Build history of the part. All positions in model axes, mm. A direction names the side the tool comes from. Give positions to 0.01 mm unless a question says otherwise; leave off trailing zeros. Loops run counter-clockwise (first coordinate to the right, second up) from the corner with the lowest first, then second, coordinate; pieces in that order, holes last. Notation, with made-up numbers: M 79,66.5 L 125,66.5 A24 ccw 125,105.5 Z; hole C 63.25,1.25 d1. An arc over 180 degrees is marked long. Put each result on its own line as item: value.
```python
from build123d import *

# Parameters (mm, degrees)
SKETCH_1_R          = 1.5
SKETCH_1_R_2        = 7.5
EXTRUDE_1_DEPTH     = 2.5
SKETCH_2_W          = 200
SKETCH_2_H          = 2.5
EXTRUDE_2_DEPTH     = 22.5
CUT_EXTRUDE_1_REACH = 327.01
SKETCH_3_R          = 1.5
CUT_EXTRUDE_2_REACH = 238.725
SKETCH_6_R          = 1.5
CUT_EXTRUDE_3_REACH = 303.968
SKETCH_7_R          = 1.5


with BuildPart() as part:
    # Эскиз1 → Бобышка-Вытянуть1 (new body)
    with BuildSketch(Plane.XY):
        Polygon((0, 0), (21, 36.373066959), (221, 36.373066959), (242, 0), (142, -173.205080757), (100, -173.205080757), align=None)
        with Locations((21.48120212, 11.846533479)):
            Circle(SKETCH_1_R, mode=Mode.SUBTRACT)
        with Locations((41.48120212, 11.846533479)):
            Circle(SKETCH_1_R, mode=Mode.SUBTRACT)
        with Locations((31.48120212, -5.473974596)):
            Circle(SKETCH_1_R, mode=Mode.SUBTRACT)
        with Locations((200.51879788, 11.846533479)):
            Circle(SKETCH_1_R, mode=Mode.SUBTRACT)
        with Locations((220.51879788, 11.846533479)):
            Circle(SKETCH_1_R, mode=Mode.SUBTRACT)
        with Locations((210.51879788, -5.473974596)):
            Circle(SKETCH_1_R, mode=Mode.SUBTRACT)
        with Locations((111, -143.204572681)):
            Circle(SKETCH_1_R, mode=Mode.SUBTRACT)
        with Locations((131, -143.204572681)):
            Circle(SKETCH_1_R, mode=Mode.SUBTRACT)
        with Locations((121, -160.525080757)):
            Circle(SKETCH_1_R, mode=Mode.SUBTRACT)
        with Locations((121, -45.610671266)):
            Circle(SKETCH_1_R_2, mode=Mode.SUBTRACT)
    extrude(amount=EXTRUDE_1_DEPTH)

    # Эскиз2 → Бобышка-Вытянуть2 (add)
    with BuildSketch(Plane(origin=(0, 0, 0), x_dir=(-1, 0, 0), z_dir=(0, 0, -1))):
        Polygon((0, 0), (2.165063509, -1.25), (-97.834936491, -174.455080757), (-100, -173.205080757), align=None)
        with Locations((-121, 37.623066959)):
            Rectangle(SKETCH_2_W, SKETCH_2_H)
        Polygon((-242, 0), (-244.165063509, -1.25), (-144.165063509, -174.455080757), (-142, -173.205080757), align=None)
    extrude(amount=-EXTRUDE_2_DEPTH)

    # Эскиз3 → Вырез-Вытянуть1 (cut, up to next)
    with BuildSketch(Plane(origin=(0, 38.873066959, 0), x_dir=(1, 0, 0), z_dir=(0, 1, 0)), mode=Mode.PRIVATE) as cut_extrude_1_sk1:
        with Locations(Location((211, -11.25, 0), (0, 0, 180))):
            Circle(SKETCH_3_R)
    cut_extrude_1_tool1 = extrude(cut_extrude_1_sk1.sketch, amount=-CUT_EXTRUDE_1_REACH, mode=Mode.PRIVATE) & part.part
    # Эскиз3 → Вырез-Вытянуть1 (cut, up to next)
    with BuildSketch(Plane(origin=(0, 38.873066959, 0), x_dir=(1, 0, 0), z_dir=(0, 1, 0)), mode=Mode.PRIVATE) as cut_extrude_1_sk2:
        with Locations(Location((201, -11.25, 0), (0, 0, 180))):
            Circle(SKETCH_3_R)
    cut_extrude_1_tool2 = extrude(cut_extrude_1_sk2.sketch, amount=-CUT_EXTRUDE_1_REACH, mode=Mode.PRIVATE) & part.part
    # Эскиз3 → Вырез-Вытянуть1 (cut, up to next)
    with BuildSketch(Plane(origin=(0, 38.873066959, 0), x_dir=(1, 0, 0), z_dir=(0, 1, 0)), mode=Mode.PRIVATE) as cut_extrude_1_sk3:
        with Locations(Location((41, -11.25, 0), (0, 0, 180))):
            Circle(SKETCH_3_R)
    cut_extrude_1_tool3 = extrude(cut_extrude_1_sk3.sketch, amount=-CUT_EXTRUDE_1_REACH, mode=Mode.PRIVATE) & part.part
    # Эскиз3 → Вырез-Вытянуть1 (cut, up to next)
    with BuildSketch(Plane(origin=(0, 38.873066959, 0), x_dir=(1, 0, 0), z_dir=(0, 1, 0)), mode=Mode.PRIVATE) as cut_extrude_1_sk4:
        with Locations(Location((31, -11.25, 0), (0, 0, 180))):
            Circle(SKETCH_3_R)
    cut_extrude_1_tool4 = extrude(cut_extrude_1_sk4.sketch, amount=-CUT_EXTRUDE_1_REACH, mode=Mode.PRIVATE) & part.part
    add(cut_extrude_1_tool1.solids().sort_by_distance((211, 38.873067, 11.25))[0], mode=Mode.SUBTRACT)
    add(cut_extrude_1_tool2.solids().sort_by_distance((201, 38.873067, 11.25))[0], mode=Mode.SUBTRACT)
    add(cut_extrude_1_tool3.solids().sort_by_distance((41, 38.873067, 11.25))[0], mode=Mode.SUBTRACT)
    add(cut_extrude_1_tool4.solids().sort_by_distance((31, 38.873067, 11.25))[0], mode=Mode.SUBTRACT)

    # Эскиз6 → Вырез-Вытянуть2 (cut, up to next)
    with BuildSketch(Plane(origin=(183.665063509, -106.039073858, 0), x_dir=(0, 0, -1), z_dir=(0.8660254037844386, -0.5000000000000003, 0)), mode=Mode.PRIVATE) as cut_extrude_2_sk1:
        with Locations(Location((-11.25, 111, 0), (0, 0, 90))):
            Circle(SKETCH_6_R)
    cut_extrude_2_tool1 = extrude(cut_extrude_2_sk1.sketch, amount=-CUT_EXTRUDE_2_REACH, mode=Mode.PRIVATE) & part.part
    # Эскиз6 → Вырез-Вытянуть2 (cut, up to next)
    with BuildSketch(Plane(origin=(183.665063509, -106.039073858, 0), x_dir=(0, 0, -1), z_dir=(0.8660254037844386, -0.5000000000000003, 0)), mode=Mode.PRIVATE) as cut_extrude_2_sk2:
        with Locations(Location((-11.25, 101, 0), (0, 0, 90))):
            Circle(SKETCH_6_R)
    cut_extrude_2_tool2 = extrude(cut_extrude_2_sk2.sketch, amount=-CUT_EXTRUDE_2_REACH, mode=Mode.PRIVATE) & part.part
    # Эскиз6 → Вырез-Вытянуть2 (cut, up to next)
    with BuildSketch(Plane(origin=(183.665063509, -106.039073858, 0), x_dir=(0, 0, -1), z_dir=(0.8660254037844386, -0.5000000000000003, 0)), mode=Mode.PRIVATE) as cut_extrude_2_sk3:
        with Locations(Location((-11.25, -59, 0), (0, 0, 90))):
            Circle(SKETCH_6_R)
    cut_extrude_2_tool3 = extrude(cut_extrude_2_sk3.sketch, amount=-CUT_EXTRUDE_2_REACH, mode=Mode.PRIVATE) & part.part
    # Эскиз6 → Вырез-Вытянуть2 (cut, up to next)
    with BuildSketch(Plane(origin=(183.665063509, -106.039073858, 0), x_dir=(0, 0, -1), z_dir=(0.8660254037844386, -0.5000000000000003, 0)), mode=Mode.PRIVATE) as cut_extrude_2_sk4:
        with Locations(Location((-11.25, -69, 0), (0, 0, 90))):
            Circle(SKETCH_6_R)
    cut_extrude_2_tool4 = extrude(cut_extrude_2_sk4.sketch, amount=-CUT_EXTRUDE_2_REACH, mode=Mode.PRIVATE) & part.part
    add(cut_extrude_2_tool1.solids().sort_by_distance((239.165064, -9.910254, 11.25))[0], mode=Mode.SUBTRACT)
    add(cut_extrude_2_tool2.solids().sort_by_distance((234.165064, -18.570508, 11.25))[0], mode=Mode.SUBTRACT)
    add(cut_extrude_2_tool3.solids().sort_by_distance((154.165064, -157.134573, 11.25))[0], mode=Mode.SUBTRACT)
    add(cut_extrude_2_tool4.solids().sort_by_distance((149.165064, -165.794827, 11.25))[0], mode=Mode.SUBTRACT)

    # Эскиз7 → Вырез-Вытянуть3 (cut, up to next)
    with BuildSketch(Plane(origin=(-2.165063509, -1.25, 0), x_dir=(0, 0, 1), z_dir=(-0.8660254037844386, -0.5000000000000003, 0)), mode=Mode.PRIVATE) as cut_extrude_3_sk1:
        with Locations(Location((11.25, -10, 0), (0, 0, 270))):
            Circle(SKETCH_7_R)
    cut_extrude_3_tool1 = extrude(cut_extrude_3_sk1.sketch, amount=-CUT_EXTRUDE_3_REACH, mode=Mode.PRIVATE) & part.part
    # Эскиз7 → Вырез-Вытянуть3 (cut, up to next)
    with BuildSketch(Plane(origin=(-2.165063509, -1.25, 0), x_dir=(0, 0, 1), z_dir=(-0.8660254037844386, -0.5000000000000003, 0)), mode=Mode.PRIVATE) as cut_extrude_3_sk2:
        with Locations(Location((11.25, -20, 0), (0, 0, 270))):
            Circle(SKETCH_7_R)
    cut_extrude_3_tool2 = extrude(cut_extrude_3_sk2.sketch, amount=-CUT_EXTRUDE_3_REACH, mode=Mode.PRIVATE) & part.part
    # Эскиз7 → Вырез-Вытянуть3 (cut, up to next)
    with BuildSketch(Plane(origin=(-2.165063509, -1.25, 0), x_dir=(0, 0, 1), z_dir=(-0.8660254037844386, -0.5000000000000003, 0)), mode=Mode.PRIVATE) as cut_extrude_3_sk3:
        with Locations(Location((11.25, -180, 0), (0, 0, 270))):
            Circle(SKETCH_7_R)
    cut_extrude_3_tool3 = extrude(cut_extrude_3_sk3.sketch, amount=-CUT_EXTRUDE_3_REACH, mode=Mode.PRIVATE) & part.part
    # Эскиз7 → Вырез-Вытянуть3 (cut, up to next)
    with BuildSketch(Plane(origin=(-2.165063509, -1.25, 0), x_dir=(0, 0, 1), z_dir=(-0.8660254037844386, -0.5000000000000003, 0)), mode=Mode.PRIVATE) as cut_extrude_3_sk4:
        with Locations(Location((11.25, -190, 0), (0, 0, 270))):
            Circle(SKETCH_7_R)
    cut_extrude_3_tool4 = extrude(cut_extrude_3_sk4.sketch, amount=-CUT_EXTRUDE_3_REACH, mode=Mode.PRIVATE) & part.part
    add(cut_extrude_3_tool1.solids().sort_by_distance((2.834936, -9.910254, 11.25))[0], mode=Mode.SUBTRACT)
    add(cut_extrude_3_tool2.solids().sort_by_distance((7.834936, -18.570508, 11.25))[0], mode=Mode.SUBTRACT)
    add(cut_extrude_3_tool3.solids().sort_by_distance((87.834936, -157.134573, 11.25))[0], mode=Mode.SUBTRACT)
    add(cut_extrude_3_tool4.solids().sort_by_distance((92.834936, -165.794827, 11.25))[0], mode=Mode.SUBTRACT)


solid = part.part
```
Q1. Slice it at B-B (x = 158.5). List the corners of the cut face in (y, z).
Here are the results:
outline: M -149.63,0 L 38.87,0 L 38.87,22.5 L 36.37,22.5 L 36.37,2.5 L -144.63,2.5 L -144.63,22.5 L -149.63,22.5 Z
Q2. Slice it at A-A (z = 19.75). List the corners of the cut face in (x, y), and give its area (3 significant figures).
Here are the results:
outline: M -2.17,-1.25 L 97.83,-174.46 L 100,-173.21 L 0,0 Z; M 21,36.37 L 221,36.37 L 221,38.87 L 21,38.87 Z; M 142,-173.21 L 144.17,-174.46 L 244.17,-1.25 L 242,0 Z
area: 1,500 mm²
Q3. Tool access for faces 1 (the flat face through (193, -87, 22.5)), 2 (the flat face through (122, 36.373, 12)), 3 (the flat face through (191.3, -87.815, 12.36)): list every direction of +Z, -Z, +X, -X, +Y, -Y with a clear straight run to the whole face (end or side of a thin tool).
Here are the results:
face 1: +Z, +X, -X, +Y, -Y
face 2: +Z, +X, -X
face 3: +Z
Q4. Slice it at D-D (y = 5). List the corners of the cut face in (x, z).
Here are the results:
outline: M 2.89,0 L 239.11,0 L 239.11,2.5 L 2.89,2.5 Z
Q5. Drop flat-ended pins along their axis: pin 1 Ø6 at (x, z) = (57.5, 8.5) entering from -Y; pin 2 Ø3.5 at (x, y) = (200.52, 11.85) entering from +Z; pin 3 Ø2.5 at (x, y) = (41.48, 11.85) entering from +Z; pin 4 Ø2.5 at (x, z) = (201, 11.25) entering from -Y. Give the stop position or say it passes through.
Here are the results:
pin 1: y = -109.79
pin 2: z = 2.5
pin 3: through
pin 4: y = -78.18
Q6. Slice it at C-C (y = -112). List the corners of the cut face in (x, z).
Here are the results:
outline: M 61.78,0 L 180.22,0 L 180.22,22.5 L 177.34,22.5 L 177.34,2.5 L 64.66,2.5 L 64.66,22.5 L 61.78,22.5 Z
Q7. Probe line 1 (Z direction, x = 31, y = 37.1); line 2 (Y direction, x = 188, z = 12.25); line 3 (Y direction, x = 93.5, z = 20.5). List the from-to ranges inside material, lowest first. Write a range as from..to.
Here are the results:
line 1: 0..9.75, 12.75..22.5
line 2: -98.53..-93.53, 36.37..38.87
line 3: -166.95..-161.95, 36.37..38.87
